Build history of the part. All positions in model axes, mm. Face numbers are marked on the shaded views. A direction names the side the tool comes from. Round coordinates to 2 decimals unless told otherwise and drop trailing zeros. Loops run counter-clockwise (first coordinate to the right, second up) from the corner with the lowest first, then second, coordinate; pieces in that order, holes last. Notation, with made-up numbers: (-24, -36) - (19, -36) arc R25 ccw to (19, 2) - close; hole circle Ø6 at (16.25, -12). An arc over 180 degrees is marked (long way). Use one line per item in the form item = value. Start each with the question number.
Q1. Saw through at C-C (z = -6.5). Give the cut face in (x, y).
Q2. Mould opens along Y. For the marked faces 3, 4, 5 and 6 say: released by +Y, released by -Y, zero draft, split by the parting line, or undercut.
Q3. Saw through at B-B (y = 15). Give the cut face in (x, z).
Q4. 3-axis set-ups, long thin cutter, end or side, ignore diameter. For the marked faces 1 and 2: which of +Z, -Z, +X, -X, +Y, -Y reach the whole face in a straight line?
Q5. Drill centre lines: line 1 (Z direction, x = 24.5, y = 0); line 2 (Z direction, x = 2, y = 15); line 3 (X direction, y = -17.5, z = 1.5). Where is each one in solid material? Low to high.
Q6. Pin check, flat tips, straight feed: pin 1 (3 mm diameter, centred on x = 19, y = -4, fed in from -Z); pin 2 (3 mm diameter, centred on y = 13, z = 9, fed in from -X); pin 3 (6 mm diameter, centred on y = -15, z = 0, fed in from +X); pin 4 (2 mm diameter, centred on x = 17, z = 7.5, fed in from +Y). Stop position of each tip, or through.
Q7. Saw through at D-D (x = 26). Give the cut face in (y, z), then the cut area to 3 significant figures.
Q8. Saw through at A-A (z = 0). Give the cut face in (x, y), then the cut area to 3 significant figures.
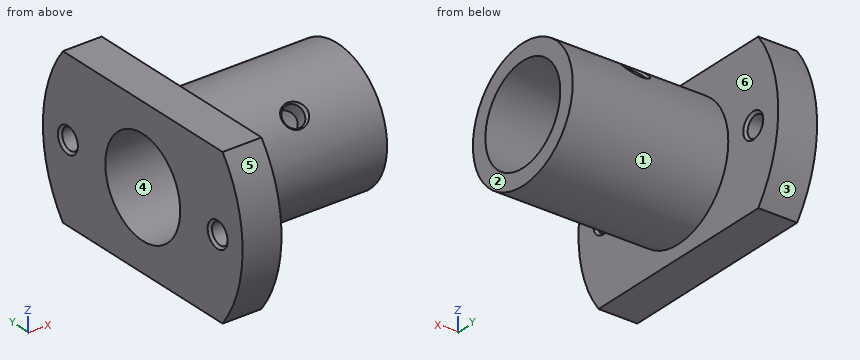
Autodesk Inventor part; units mm, degrees
ref_plane "to_screw1_XY" through (18, -5.3033, 5.3033) normal (0, -0.7071, 0.7071) x (1, 0, 0)
ref_plane "to_screw1_YZ" through (18, -5.3033, 5.3033) normal (1, 0, 0) x (0, 0.7071, 0.7071)
ref_plane "to_screw1_ZX" through (18, -5.3033, 5.3033) normal (0, 0.7071, 0.7071) x (0, -0.7071, 0.7071)
sketch "Sketch_1" plane through (0, 0, 0) normal (0, 0, 1) x (1, 0, 0)
  line L0 (30, 0) -> (0, 0)
  line L1 (0, 20) -> (0, 7.5)
  line L2 (0, 7.5) -> (30, 7.5)
  line L3 (30, 7.5) -> (30, 10)
  line L4 (30, 10) -> (6, 10)
  line L5 (6, 10) -> (6, 20)
  line L6 (6, 20) -> (0, 20)
revolve "Revolution1" add sketch "Sketch_1" angle 360 about axis through (30, 0, 0) along (1, 0, 0)
sketch "Sketch_3" plane through (0, 0, 0) normal (0, -0.7071, 0.7071) x (1, 0, 0)
  line L0 (18, 7.2284) -> (18, 10)
  line L1 (18, 10) -> (20, 10)
  line L2 (20, 10) -> (19.621, 9.621)
  line L3 (19.621, 9.621) -> (19.621, 7.2284)
  line L4 (19.621, 7.2284) -> (18, 7.2284)
  line L5 (18, 7.2284) -> (18, 10)
revolve "Revolution2" cut sketch "Sketch_3" angle 360 about axis through (18, 5.1113, 5.1113) along (0, -0.7071, -0.7071)
thread "Thread1"
sketch "Sketch_2" plane through (0, 0, 0) normal (0, -0.7071, -0.7071) x (1, 0, 0)
  line L0 (18, 7.2284) -> (18, 10)
  line L1 (18, 10) -> (20, 10)
  line L2 (20, 10) -> (19.621, 9.621)
  line L3 (19.621, 9.621) -> (19.621, 7.2284)
  line L4 (19.621, 7.2284) -> (18, 7.2284)
  line L5 (18, 7.2284) -> (18, 10)
revolve "Revolution3" cut sketch "Sketch_2" angle 360 about axis through (18, -5.1113, 5.1113) along (0, 0.7071, -0.7071)
thread "Thread2"
sketch "Sketch_4" plane through (0, 0, 0) normal (1, 0, 0) x (0, 1, 0)
  circle A0 centre (0, 0) radius 150
  line L0 (-50, 12) -> (-50, -12)
  line L1 (-50, -12) -> (50, -12)
  line L2 (50, -12) -> (50, 12)
  line L3 (50, 12) -> (-50, 12)
extrude "Extrusion1" cut sketch "Sketch_4" along normal blind 30
sketch "Sketch_12" plane through (0, 0, 0) normal (0, 0, 1) x (1, 0, 0)
  line L0 (6, 15) -> (0, 15)
  line L1 (0, 15) -> (0, 17)
  line L2 (0, 17) -> (0.379, 16.621)
  line L3 (0.379, 16.621) -> (5.621, 16.621)
  line L4 (5.621, 16.621) -> (6, 17)
  line L5 (6, 17) -> (6, 15)
  line L6 (6, 15) -> (0, 15)
revolve "Revolution4" cut sketch "Sketch_12" angle 360 about axis through (6, 15, 0) along (1, 0, 0)
thread "Thread3"
sketch "Sketch_14" plane through (0, 0, 0) normal (0, 0, 1) x (1, 0, 0)
  line L0 (0, -15) -> (6, -15)
  line L1 (6, -15) -> (6, -17)
  line L2 (6, -17) -> (5.621, -16.621)
  line L3 (5.621, -16.621) -> (0.379, -16.621)
  line L4 (0.379, -16.621) -> (0, -17)
  line L5 (0, -17) -> (0, -15)
  line L6 (0, -15) -> (6, -15)
revolve "Revolution5" cut sketch "Sketch_14" angle 360 about axis through (0, -15, 0) along (-1, 0, 0)
thread "Thread4"
ref_plane "to_screw1_XY" through (18, -5.3033, 5.3033) normal (0, -0.7071, 0.7071) x (1, 0, 0)
ref_plane "to_screw1_YZ" through (18, -5.3033, 5.3033) normal (1, 0, 0) x (0, 0.7071, 0.7071)
ref_plane "to_screw1_ZX" through (18, -5.3033, 5.3033) normal (0, 0.7071, 0.7071) x (0, -0.7071, 0.7071)
ref_plane "to_screw2_XY" through (18, 5.3033, 5.3033) normal (0, 0.7071, 0.7071) x (1, 0, 0)
ref_plane "to_screw2_YZ" through (18, 5.3033, 5.3033) normal (1, 0, 0) x (0, 0.7071, -0.7071)
ref_plane "to_screw2_ZX" through (18, 5.3033, 5.3033) normal (0, 0.7071, -0.7071) x (0, 0.7071, 0.7071)
properties part number "STHCBT15-MB_ss"
Report:
q1.outline = (0, -18.91) - (6, -18.91) - (6, -7.6) - (30, -7.6) - (30, -3.74) - (0, -3.74) - close; (0, 3.74) - (30, 3.74) - (30, 7.6) - (6, 7.6) - (6, 18.91) - (0, 18.91) - close
q2.face_3 = released by +Y
q2.face_4 = undercut
q2.face_5 = released by -Y
q2.face_6 = zero draft
q3.outline = (0, -12) - (6, -12) - (6, -2) - (5.62, -1.62) - (0.38, -1.62) - (0, -2) - close; (0, 2) - (0.38, 1.62) - (5.62, 1.62) - (6, 2) - (6, 12) - (0, 12) - close
q4.face_1 = +X
q4.face_2 = +Z, -Z, +X, +Y, -Y
q5.line_1 = -10 to -7.5, 7.5 to 10
q5.line_2 = -12 to -1.62, 1.62 to 12
q5.line_3 = 0 to 6
q6.pin_1 = -9.68
q6.pin_2 = 0
q6.pin_3 = 6
q6.pin_4 = 6.96
q7.outline = circle Ø20 at (0, 0); hole circle Ø15 at (0, 0)
q7.area = 137 mm²
q8.outline = (0, -20) - (6, -20) - (6, -17) - (5.62, -16.62) - (0.38, -16.62) - (0, -17) - close; (0, -13) - (0.38, -13.38) - (5.62, -13.38) - (6, -13) - (6, -10) - (30, -10) - (30, -7.5) - (0, -7.5) - close; (0, 7.5) - (30, 7.5) - (30, 10) - (6, 10) - (6, 13) - (5.62, 13.38) - (0.38, 13.38) - (0, 13) - close; (0, 17) - (0.38, 16.62) - (5.62, 16.62) - (6, 17) - (6, 20) - (0, 20) - close
q8.area = 231 mm²
